Input: part model. Units: mm. Frame: model coordinates. Round coordinates to 2 decimals unless told otherwise and drop trailing zeros. Loops run counter-clockwise (first coordinate to the right, second up) from the corner with the lowest first, then second, coordinate; pieces in that order, holes last.
(1) Line query: line 1 (X direction, y = 0.4, z = -24.5); line 2 (X direction, y = 3, z = 15); line 3 (X direction, y = 1.25, z = -0.5). Output: solid intervals per line, ascending.
(2) Cut plane C-C, the plane z = -13.5. Output: boundary loops of the cut face in (x, y) (3 decimals).
(3) Cut plane D-D, the plane x = 27. Output: boundary loops of the cut face in (y, z) (3 decimals), and give its area (3 significant figures).
(4) Cut plane A-A, the plane x = 0. Output: boundary loops of the cut face in (y, z) (3 decimals).
(5) Cut plane B-B, the plane z = 0. Output: boundary loops of the cut face in (x, y) (3 decimals).
from build123d import *

# Parameters (mm, degrees)
SKETCH1_R                   = 34.925
SKETCH1_R_2                 = 12.7
SKETCH1_R_3                 = 3.429
BOSS_EXTRUDE1_DEPTH         = 3.175
TAP_DRILL_FOR_2_HELICOIL1_D = 2.38252
CIRPATTERN1_COUNT           = 6


with BuildPart() as part:
    # Sketch1 → Boss-Extrude1 (new body)
    with BuildSketch(Plane(origin=(0, 0, 0), x_dir=(1, 0, 0), z_dir=(0, 1, 0))):
        with Locations(Location((0, 0, 0), (0, 0, 270))):
            Circle(SKETCH1_R)
        with Locations(Location((0, 0, 0), (0, 0, 270))):
            Circle(SKETCH1_R_2, mode=Mode.SUBTRACT)
        with Locations(Location((0, 29.3624, 0), (0, 0, 270))):
            Circle(SKETCH1_R_3, mode=Mode.SUBTRACT)
        with Locations(Location((25.428584316, 14.6812, 0), (0, 0, 270))):
            Circle(SKETCH1_R_3, mode=Mode.SUBTRACT)
        with Locations(Location((25.428584316, -14.6812, 0), (0, 0, 270))):
            Circle(SKETCH1_R_3, mode=Mode.SUBTRACT)
        with Locations(Location((0, -29.3624, 0), (0, 0, 270))):
            Circle(SKETCH1_R_3, mode=Mode.SUBTRACT)
        with Locations(Location((-25.428584316, -14.6812, 0), (0, 0, 270))):
            Circle(SKETCH1_R_3, mode=Mode.SUBTRACT)
        with Locations(Location((-25.428584316, 14.6812, 0), (0, 0, 270))):
            Circle(SKETCH1_R_3, mode=Mode.SUBTRACT)
    extrude(amount=BOSS_EXTRUDE1_DEPTH)

    # Tap Drill for #2 Helicoil1 (through all)
    with Locations(Plane(origin=(0, 0, 0), x_dir=(-1, 0, 0), z_dir=(0, -1, 0))):
        with Locations((14.6812, 25.428584316)):
            tap_drill_for_2_helicoil1 = Hole(TAP_DRILL_FOR_2_HELICOIL1_D / 2)

    # CirPattern1: Tap Drill for #2 Helicoil1 ×6 about axis
    cirpattern1_axis = Axis((0, 0, 0), (0, 1, 0))
    for i in range(1, CIRPATTERN1_COUNT):
        add(tap_drill_for_2_helicoil1.rotate(cirpattern1_axis, i * 360 / CIRPATTERN1_COUNT), mode=Mode.SUBTRACT)


solid = part.part
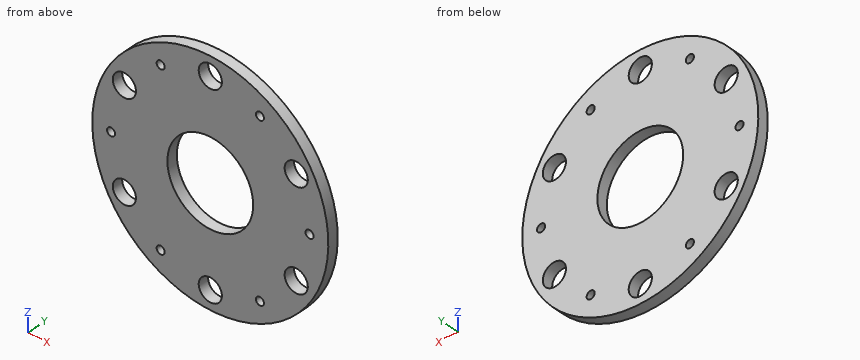
Reported:
1. line 1: x = -24.89 to -15.43, -13.93 to 13.93, 15.43 to 24.89
1. line 2: x = -31.54 to -28.84, -22.01 to 22.01, 28.84 to 31.54
1. line 3: x = -34.92 to -30.44, -28.28 to -12.69, 12.69 to 28.28, 30.44 to 34.92
2. outline: (-32.21, 0) - (-28.648, 0) - (-28.648, 3.175) - (-32.21, 3.175) - close; (-22.209, 0) - (22.209, 0) - (22.209, 3.175) - (-22.209, 3.175) - close; (28.648, 0) - (32.21, 0) - (32.21, 3.175) - (28.648, 3.175) - close
3. outline: (0, -22.153) - (3.175, -22.153) - (3.175, -17.729) - (0, -17.729) - close; (0, -11.633) - (3.175, -11.633) - (3.175, 11.633) - (0, 11.633) - close; (0, 17.729) - (3.175, 17.729) - (3.175, 22.153) - (0, 22.153) - close
3. area: 102 mm2
4. outline: (0, -34.925) - (3.175, -34.925) - (3.175, -32.791) - (0, -32.791) - close; (0, -25.933) - (3.175, -25.933) - (3.175, -12.7) - (0, -12.7) - close; (0, 12.7) - (3.175, 12.7) - (3.175, 25.933) - (0, 25.933) - close; (0, 32.791) - (3.175, 32.791) - (3.175, 34.925) - (0, 34.925) - close
5. outline: (-34.925, 0) - (-30.554, 0) - (-30.554, 3.175) - (-34.925, 3.175) - close; (-28.171, 0) - (-12.7, 0) - (-12.7, 3.175) - (-28.171, 3.175) - close; (12.7, 0) - (28.171, 0) - (28.171, 3.175) - (12.7, 3.175) - close; (30.554, 0) - (34.925, 0) - (34.925, 3.175) - (30.554, 3.175) - close
